```python
from build123d import *

# Parameters (mm, degrees)
CYLINDER003_R     = 2.5
CYLINDER003_DEPTH = 23
CYLINDER002_R     = 2.5
CYLINDER002_DEPTH = 23
BOX_W             = 59.5
BOX_H             = 35
BOX_DEPTH         = 23
CYLINDER001_R     = 17.5
CYLINDER001_DEPTH = 23
CYLINDER_R        = 42.5
CYLINDER_DEPTH    = 23
CHAMFER_SIZE2     = 1
CHAMFER_SIZE      = 10


with BuildPart() as cylinder003:
    # Cylinder003 → Cylinder003 (new body)
    with BuildSketch(Plane(origin=(0, -30, 0), x_dir=(1, 0, 0), z_dir=(0, 0, 1))):
        Circle(CYLINDER003_R)
    extrude(amount=CYLINDER003_DEPTH)


with BuildPart() as cylinder002:
    # Cylinder002 → Cylinder002 (new body)
    with BuildSketch(Plane(origin=(0, 30, 0), x_dir=(1, 0, 0), z_dir=(0, 0, 1))):
        Circle(CYLINDER002_R)
    extrude(amount=CYLINDER002_DEPTH)


with BuildPart() as cube:
    # Box → Box (new body)
    with BuildSketch(Plane(origin=(-42.5, -17.5, 0), x_dir=(1, 0, 0), z_dir=(0, 0, 1))):
        with Locations((29.75, 17.5)):
            Rectangle(BOX_W, BOX_H)
    extrude(amount=BOX_DEPTH)


with BuildPart() as cylinder001:
    # Cylinder001 → Cylinder001 (new body)
    with BuildSketch(Plane(origin=(17, 0, 0), x_dir=(1, 0, 0), z_dir=(0, 0, 1))):
        Circle(CYLINDER001_R)
    extrude(amount=CYLINDER001_DEPTH)


with BuildPart() as cut003:
    # Cylinder → Cylinder (new body)
    with BuildSketch(Plane.XY):
        Circle(CYLINDER_R)
    extrude(amount=CYLINDER_DEPTH)

    # Chamfer
    chamfer_edges = [cut003.edges().sort_by_distance(p)[0] for p in [
        (-42.5, 0, 23),
    ]]
    chamfer_side = cut003.faces().sort_by_distance((-42.5, 0, 11.5))[0]
    chamfer(chamfer_edges, length=CHAMFER_SIZE, length2=CHAMFER_SIZE2, reference=chamfer_side)

    # Cut: cut Cylinder001
    add(cylinder001.part, mode=Mode.SUBTRACT)

    # Cut001: cut Cube
    add(cube.part, mode=Mode.SUBTRACT)

    # Cut002: cut Cylinder002
    add(cylinder002.part, mode=Mode.SUBTRACT)

    # Cut003: cut Cylinder003
    add(cylinder003.part, mode=Mode.SUBTRACT)


solid = cut003.part
```
The listing builds one solid part. Answer for the finished solid, in the listing's coordinates (mm). A direction names the side the tool comes from. Coordinates: 2 decimals unless noted, no trailing zeros. Loops run counter-clockwise (first coordinate to the right, second up) from the corner with the lowest first, then second, coordinate; pieces in that order, holes last. Notation, with made-up numbers: M -25,48 L 7,48 A13 ccw 7,55 Z; hole C 72.5,-13 d8. An arc over 180 degrees is marked long. Answer as a JSON object with one key per item and string values. Group by question number.
Item 1: Which of the six approach directions +Z, -Z, +X, -X, +Y, -Y give full straight-line access (tool end or side, diameter ignored) to faces 1 (the face through (-11, -17.5, 11)), 2 (the face through (41.63, -1.58, 21.4))?
Item 2: Consider L1, parallel to Y at x = 0, z = 12.5; L2, parallel to Y at x = 0, z = 14; L3, parallel to Y at x = 8, z = 15.5. Determine where each line is inside the solid, lowest interval first.
Item 3: Each of these flat-tipped pins is pushed along its axis until it touches: P1, Ø5, axis at x = -28.5, z = 5.5, coming from the +Y side; P2, Ø8, axis at y = 7, z = 9.5, coming from the +X side; P3, Ø5, axis at x = -1, z = 10, coming from the -Y side. Where does it stop, or does it pass through?
Item 4: Section C-C (y = 0) is taken. Write down the section's boundary in (x, z).
Item 5: Section A-A (x = 0) is taken. Write down the section's boundary in (y, z).
Item 6: Determine the mould class of faces 3 (the face through (1, -18, 0)), 4 (the face through (34.496, -0.385, 11.339)), 5 (the face through (42.47, -1.62, 6.41)) for opening direction Y: +Y half, -Y half, draft (parallel to the pull), parting line (faces both ways), or undercut.
Item 7: Section B-B (z = 12) is taken. Write down the section's boundary in (x, y), and give its area (3 significant figures).
Solved:
{
 "1": {"face 1": "+Z, -Z, -X", "face 2": "+Z"},
 "2": {"L1": "y = -42.5 to -32.5, -27.5 to -17.5, 17.5 to 27.5, 32.5 to 42.5", "L2": "y = -42.4 to -32.5, -27.5 to -17.5, 17.5 to 27.5, 32.5 to 42.4", "L3": "y = -41.49 to -17.5, 17.5 to 41.49"},
 "3": {"P1": "stops at y = 33.62", "P2": "stops at x = 42.39", "P3": "stops at y = -42.5"},
 "4": {"outline": "M 34.5,0 L 42.5,0 L 42.5,13 L 41.5,23 L 34.5,23 Z"},
 "5": {"outline": "M -42.5,0 L -32.5,0 L -32.5,23 L -41.5,23 L -42.5,13 Z; M -27.5,0 L -17.5,0 L -17.5,23 L -27.5,23 Z; M 17.5,0 L 27.5,0 L 27.5,23 L 17.5,23 Z; M 32.5,0 L 42.5,0 L 42.5,13 L 41.5,23 L 32.5,23 Z"},
 "6": {"face 3": "draft", "face 4": "undercut", "face 5": "parting line"},
 "7": {"outline": "M -38.73,-17.5 A42.5 ccw long -38.73,17.5 L 17,17.5 A17.5 cw 17,-17.5 Z; hole C 0,-30 d5; hole C 0,30 d5", "area": "3,110 mm2"}
}
